Job drawing, mm, ordinate dimensions from the low corner. One solid piece. Round coordinates to 2 decimals unless told otherwise and drop trailing zeros. Write each loop counter-clockwise with the first axis right and the second up, starting at its lowest first coordinate (ties: lowest second). Pieces come first, ordered by that corner, then holes. Notation, with made-up numbers: M 40.5,-0.75 L 66.5,-0.75 A22 cw 66.5,23.25 Z; hole C 76,2 d2. An arc over 180 degrees is marked long. One line per item, written item: value. Start each with the question number.
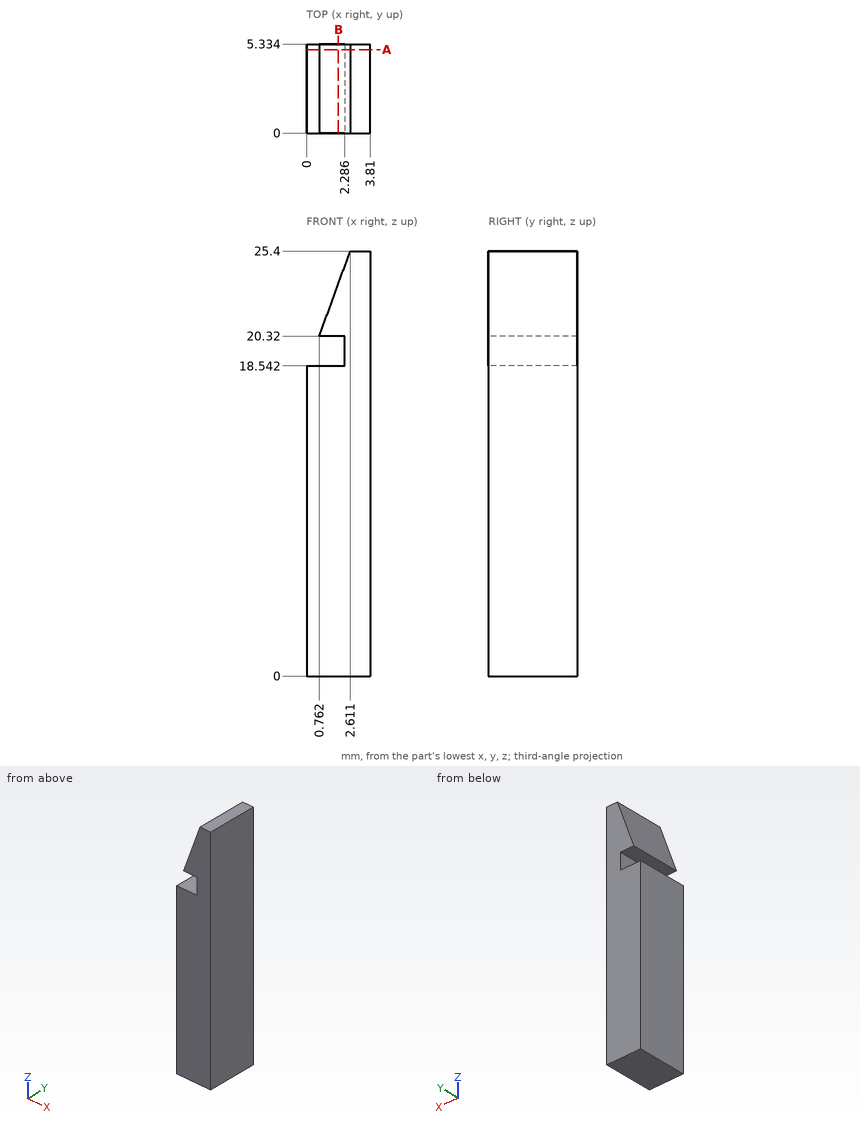
Item 1: Cut at B-B, the plane x = 1.9. Write the cut outline in (y, z).
Item 2: Cut at A-A, the plane y = 5. Write the cut outline in (x, z), plus the area to 3 significant figures.
Item 3: Drill centre lines: line 1 (Z direction, x = 0.2, y = 0.45); line 2 (X direction, y = 4.7, z = 20); line 3 (X direction, y = 2.2, z = 20.5). Where is each one in solid material? Low to high.
Item 4: Drop flat-ended pins along their axis: pin 1 (1.4 mm diameter, centred on y = 2, z = 19.5, fed in from -X); pin 2 (2 mm diameter, centred on x = 2, z = 21, fed in from -Y). Give the stop position or say it passes through.
Computed values:
1. outline: M 0,0 L 5.33,0 L 5.33,18.54 L 0,18.54 Z; M 0,20.32 L 5.33,20.32 L 5.33,23.45 L 0,23.45 Z
2. outline: M 0,0 L 3.81,0 L 3.81,25.4 L 2.61,25.4 L 0.76,20.32 L 2.29,20.32 L 2.29,18.54 L 0,18.54 Z
2. area: 84.1 mm2
3. line 1: z = 0 to 18.54
3. line 2: x = 2.29 to 3.81
3. line 3: x = 0.83 to 3.81
4. pin 1: stops at x = 2.29
4. pin 2: stops at y = 0
